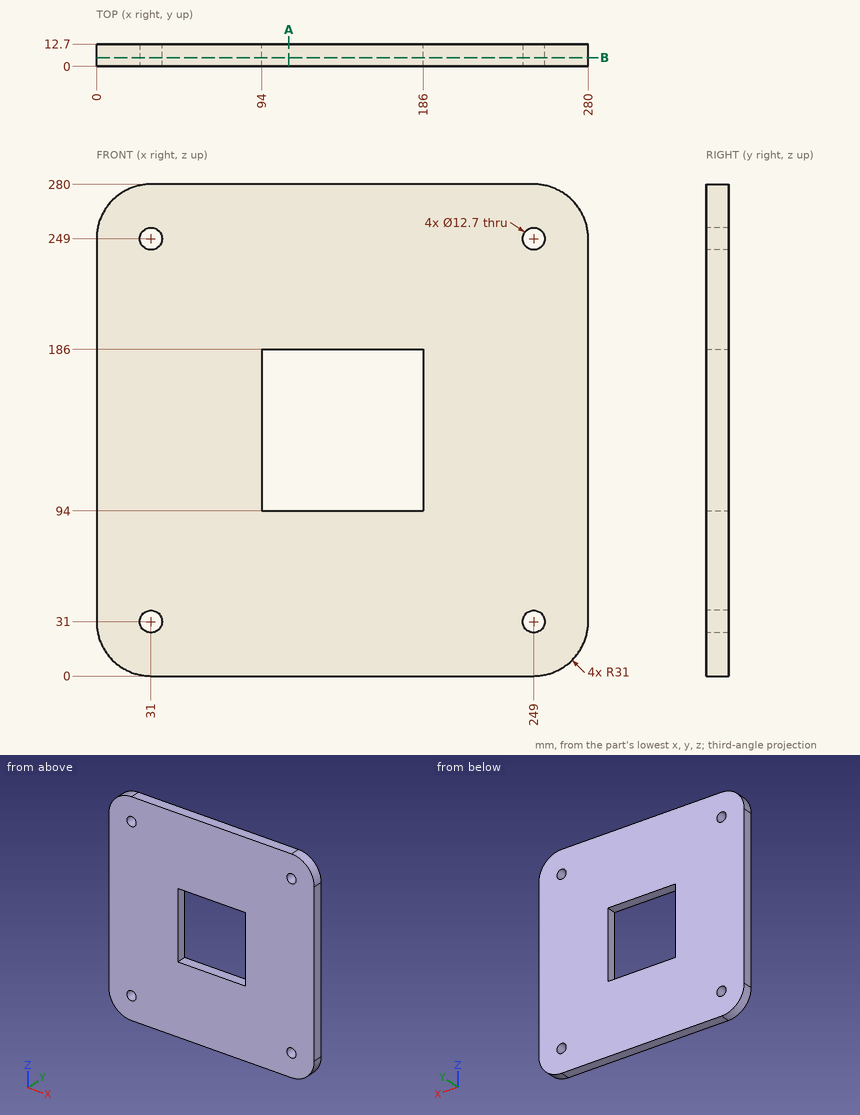
Geometry: see drawing. Coordinates: mm, zero at the bounding-box minimum. Round coordinates to 2 decimals unless told otherwise and drop trailing zeros. Write each loop counter-clockwise with the first axis right and the second up, starting at its lowest first coordinate (ties: lowest second). Pieces come first, ordered by that corner, then holes.
1) Cut plane A-A (x = 109.5). Return the cut outline in (y, z).
2) Ray query, L1, parallel to X at y = 7.25, z = 31; L2, parallel to Z at x = 28, y = 8.75. Return the intervals inside material, ascending.
3) Cut plane B-B (y = 5). Return the cut outline in (x, z).
Geometry says:
1. outline: (0, 0) - (12.7, 0) - (12.7, 94) - (0, 94) - close; (0, 186) - (12.7, 186) - (12.7, 280) - (0, 280) - close
2. L1: x = 0 to 24.65, 37.35 to 242.65, 255.35 to 280
2. L2: z = 0.15 to 25.4, 36.6 to 243.4, 254.6 to 279.85
3. outline: (0, 31) arc R31 ccw to (31, 0) - (249, 0) arc R31 ccw to (280, 31) - (280, 249) arc R31 ccw to (249, 280) - (31, 280) arc R31 ccw to (0, 249) - close; hole circle Ø12.7 at (31, 31); hole circle Ø12.7 at (31, 249); hole (94, 94) - (186, 94) - (186, 186) - (94, 186) - close; hole circle Ø12.7 at (249, 31); hole circle Ø12.7 at (249, 249)
